The figure shows three views and two pictorial views of one solid part (mm, origin at its lowest corner). Answer the questions. Coordinates: 2 decimals unless noted, no trailing zeros. Order: outer loops, then holes, each group sorted by start corner. A loop starts at its lowest first (then second) coordinate and runs counter-clockwise, first axis right, second up.
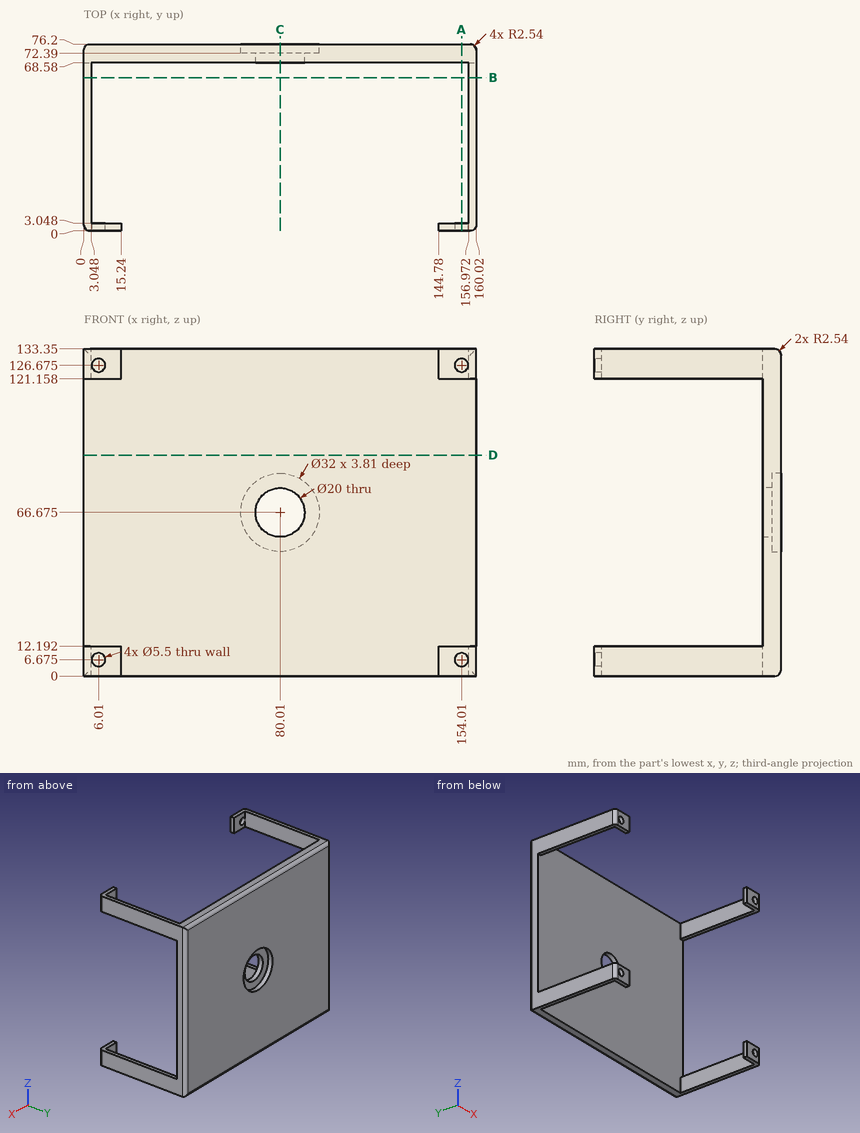
Q1. The part is cut by section A-A, the plane x = 154.01. Determine the outline of the cut face in (y, z) (3 decimals), then the cut area to 3 significant figures.
Q2. The part is cut by section C-C, the plane x = 80.01. Determine the outline of the cut face in (y, z) (3 decimals), then the cut area to 3 significant figures.
Q3. The part is cut by section D-D, the plane z = 90. Determine the outline of the cut face in (x, y).
Q4. Each of these flat-tipped pins is pushed along its axis until it touches: P1, Ø12, axis at x = 75, z = 98, coming from the -Y side; P2, Ø1.5, axis at y = 1.5, z = 7, coming from the -X side; P3, Ø0.9, axis at y = 1, z = 128.5, coming from the +X side. Where does it stop, or does it pass through?
Q5. Straight lines are drawn through the part: L1, parallel to X at y = 19, z = 127; L2, parallel to Z at x = 154.01, y = 2.45 (3 decimals); L3, parallel to Y at x = 153, z = 96.5. For each, find the intervals that lie inside material, in ascending order.
Q6. The part is cut by section B-B, the plane y = 62.5. Determine the outline of the cut face in (x, z), then the cut area to 3 significant figures.
Computed values:
1. outline: (0, 0) - (3.048, 0) - (3.048, 3.925) - (0, 3.925) - close; (0, 9.425) - (3.048, 9.425) - (3.048, 12.192) - (0, 12.192) - close; (0, 121.158) - (3.048, 121.158) - (3.048, 123.925) - (0, 123.925) - close; (0, 129.425) - (3.048, 129.425) - (3.048, 133.35) - (0, 133.35) - close; (68.58, 0) - (73.66, 0) arc R2.54 ccw to (76.2, 2.54) - (76.2, 130.81) arc R2.54 ccw to (73.66, 133.35) - (68.58, 133.35) - close
1. area: 1,050 mm2
2. outline: (68.58, 0) - (73.66, 0) arc R2.54 ccw to (76.2, 2.54) - (76.2, 50.675) - (72.39, 50.675) - (72.39, 56.675) - (68.58, 56.675) - close; (68.58, 76.675) - (72.39, 76.675) - (72.39, 82.675) - (76.2, 82.675) - (76.2, 130.81) arc R2.54 ccw to (73.66, 133.35) - (68.58, 133.35) - close
2. area: 815 mm2
3. outline: (0, 68.58) - (160.02, 68.58) - (160.02, 73.66) arc R2.54 ccw to (157.48, 76.2) - (2.54, 76.2) arc R2.54 ccw to (0, 73.66) - close
4. P1: stops at y = 68.58
4. P2: stops at x = 0.02
4. P3: stops at x = 159.77
5. L1: x = 0 to 3.05, 156.97 to 160.02
5. L2: z = 0 to 3.925, 9.425 to 12.192, 121.158 to 123.925, 129.425 to 133.35
5. L3: y = 68.58 to 76.2
6. outline: (0, 0) - (3.05, 0) - (3.05, 12.19) - (0, 12.19) - close; (0, 121.16) - (3.05, 121.16) - (3.05, 133.35) - (0, 133.35) - close; (156.97, 0) - (160.02, 0) - (160.02, 12.19) - (156.97, 12.19) - close; (156.97, 121.16) - (160.02, 121.16) - (160.02, 133.35) - (156.97, 133.35) - close
6. area: 149 mm2
